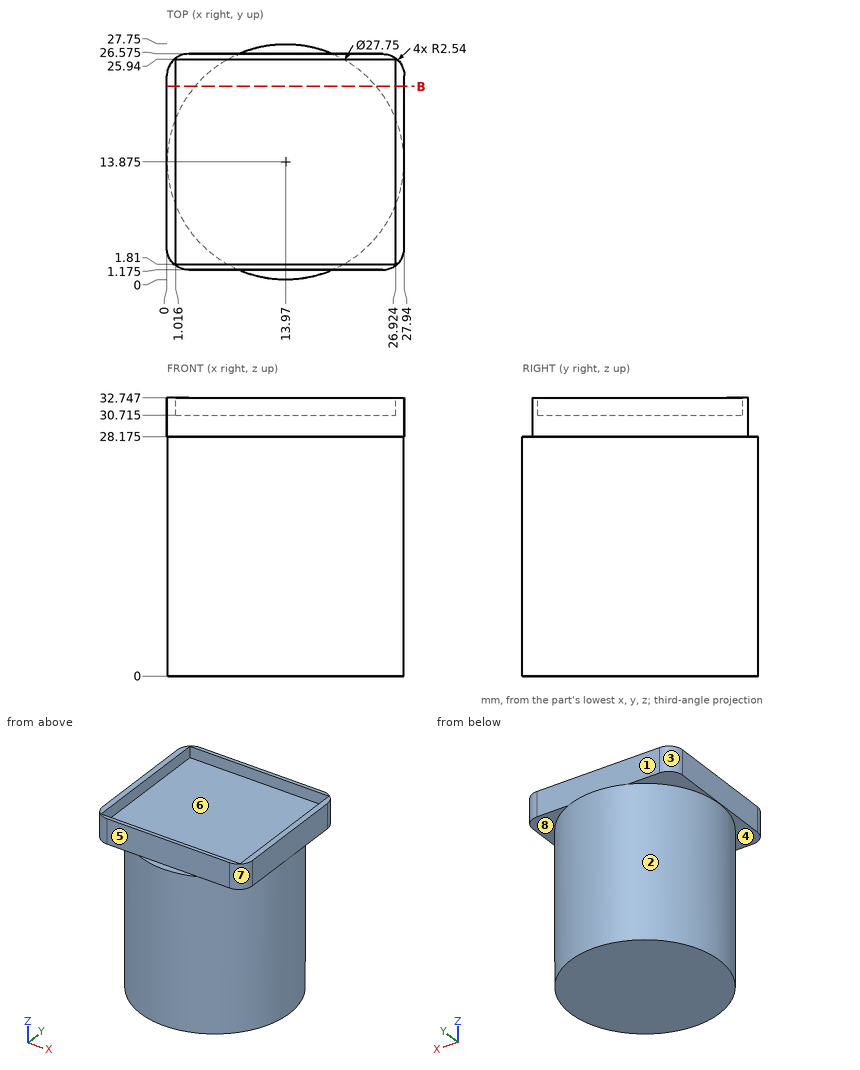
The drawing under review shows one solid part. Ordinate dimensions are in mm from its lowest x, y, z. A direction names the side the tool comes from. Give positions to 0.01 mm unless a question says otherwise; leave off trailing zeros. Write each loop counter-clockwise with the first axis right and the second up, starting at its lowest first coordinate (ties: lowest second). Pieces come first, ordered by that corner, then holes. Notation, with made-up numbers: (26.5, 20) -> (59.5, 20) arc R21 ccw to (59.5, 47) -> close; hole circle Ø3 at (60, -23). An arc over 180 degrees is marked (long way). Use CSV: the item, a comma, the result in double quotes.
Q1. Tool access review of the marked faces 1, 2, 3, 4 and 5: name each direction out of +Z, -Z, +X, -X, +Y, -Y from which nothing blocks a thin tool from reaching the whole face with its end or side.
Conclusion:
face 1,"+Z, +X, -X, +Y"
face 2,"-Z"
face 3,"+Z, -Z, -X, +Y"
face 4,"-Z, -X"
face 5,"+Z, +X, -X, -Y"
Q2. Take a section at B-B, the plane y = 22.75. Write out the cut boundary in (x, z) (1 decimal), then the cut area to 3 significant figures.
Conclusion:
outline,"(0, 28.2) -> (3.3, 28.2) -> (3.3, 0) -> (24.6, 0) -> (24.6, 28.2) -> (27.9, 28.2) -> (27.9, 32.7) -> (26.9, 32.7) -> (26.9, 30.7) -> (1, 30.7) -> (1, 32.7) -> (0, 32.7) -> close"
area,"676 mm2"
Q3. Mouldability with a two-part tool opening along Y and no side actions: class the marked faces 6, 7 and 8 as pulls with the +Y half, pulls with the -Y half, needs draft (parallel to the pull), parting line crosses it, or undercut.
Conclusion:
face 6,"undercut"
face 7,"pulls with the -Y half"
face 8,"needs draft"
Q4. To check wall thickness, follow probe 1 along Z at (x, y) = (3.5, 11.5) (1 decimal); probe 2 along Y at (x, z) = (2.75, 29) (1 decimal); probe 3 along Z at (x, y) = (22.5, 25) (1 decimal). State the ranges of each line that lie inside material, in increasing order. Write a range as [from, to].
Conclusion:
probe 1,"[0, 30.7]"
probe 2,"[1.2, 26.6]"
probe 3,"[28.2, 30.7]"
Q5. For P1, Ø6.5, axis at x = 23, y = 10.5, coming from the -Z side; P2, Ø1, axis at x = 19, z = 32, coming from the -Y side (1 decimal); P3, Ø0.6, axis at x = 12, y = 27, coming from the +Z side (1 decimal); P4, Ø5, axis at y = 24, z = 3.5, coming from the -X side, all flat-tipped, find the tip position at first contact; note any pin that passes through.
Conclusion:
P1,"z = 0"
P2,"y = 1.2"
P3,"z = 28.2"
P4,"x = 2.38"
